Can you work these out from the model? Positions are in its coordinate system, mm. A direction names the side the tool comes from. Round coordinates to 2 decimals unless told otherwise and drop trailing zeros. Order: outer loops, then holes, each group sorted by start corner. A loop starts at its lowest first (then second) coordinate and runs counter-clockwise, first axis right, second up. Notation, with made-up numbers: M 89,-37 L 131,-37 A30 cw 131,-6 Z; hole C 55.5,5.25 d8. An arc over 180 degrees is marked long. Answer as a JSON object with one key per item and string values. Group by question number.
Autodesk Inventor part; units mm, degrees
ref_plane "Work Plane1" through (0, -29, 0) normal (0, 1, 0) x (-1, 0, 0)
ref_plane "Work Plane2" through (-18.485, -29, 0) normal (0, 0, 1) x (1, 0, 0)
ref_plane "YZ Plane" through (0, 0, 0) normal (1, 0, 0) x (0, 1, 0)
sketch "Sketch1" plane through (0, 0, 0) normal (0, 0, 1) x (1, 0, 0)
  circle A0 centre (0, 0) radius 28 construction
  circle A1 centre (0, 0) radius 29 construction
  circle A2 centre (0, 0) radius 28
  circle A3 centre (0, 0) radius 29
  line L0 (0, 0) -> (27.8935, 2.4404)
  line L1 (0, 0) -> (28, 0) construction
  line L2 (0, 0) -> (0, -29.5121)
  line L3 (0, -28) -> (0, -29)
  line L4 (27.8935, 2.4404) -> (28.8971, 2.4404)
  dimension "d0" = 56
  dimension "d1" = 58
  dimension "d2" = 5
revolve "Revolution1" add sketch "Sketch1" angle 360 about axis through (0, 0, 0) along (0, -1, 0) picked at (16.0405, -23.5642) contours A2 L4 A3 L2
sketch "Sketch2" plane through (0, 2.4404, 0) normal (0, 1, 0) x (1, 0, 0)
  line L0 (-0.5, -30) -> (0.5, -30)
  line L1 (0.5, -30) -> (0.5, 30)
  line L2 (0.5, 30) -> (-0.5, 30)
  line L3 (-0.5, 30) -> (-0.5, -30)
  line L4 (-0.5, -30) -> (0.5, 30) construction
  line L5 (0.5, -30) -> (-0.5, 30) construction
  line L6 (30, -0.5) -> (-30, -0.5)
  line L7 (-30, -0.5) -> (-30, 0.5)
  line L8 (-30, 0.5) -> (30, 0.5)
  line L9 (30, 0.5) -> (30, -0.5)
  circle A0 centre (0, 0) radius 28.8971
  line L10 (30, -0.5) -> (-30, 0.5) construction
  line L11 (-30, -0.5) -> (30, 0.5) construction
  point P0 (0.5, 0.5)
  point P1 (-0.5, 0.5)
  point P2 (-0.5, -0.5)
  point P3 (0.5, -0.5)
  dimension "d4" = 1
  dimension "d5" = 60
  dimension "d6" = 60
  dimension "d7" = 1
extrude "Extrusion1" cut sketch "Sketch2" against normal blind 15 contours L3 A0 L1 L0 | L3 L6 L1 A0 | L6 A0 L8 L3 | L3 L8 L1 L6 | L6 L7 L8 A0 | L1 L8 A0 L6 | A0 L8 L9 L6 | L3 A0 L1 L8 | L3 L2 L1 A0
ref_plane "Work Plane1" through (0, -29, 0) normal (0, 1, 0) x (-1, 0, 0)
sketch "Sketch3" plane through (0, -29, 0) normal (0, 1, 0) x (-1, 0, 0)
  arc A0 (-0.5, 28.8928) -> (-28.8928, 0.5) centre (0, 0) ccw
  arc A1 (-0.5, -26.1344) -> (0.5, -26.1344) centre (0, 0) ccw
  line L0 (0.5, -25.0201) -> (0.5, -26.1344)
  arc A2 (-0.5, -25.0201) -> (0.5, -25.0201) centre (0, 0) ccw
  line L1 (-0.5, -26.1344) -> (-0.5, -25.0201)
  circle A3 centre (0, 0) radius 26.1392
  line L2 (18.485, 18.4813) -> (-18.485, 18.4813)
  line L3 (-18.485, 18.4813) -> (-18.485, -18.4813)
  line L4 (-18.485, -18.4813) -> (18.485, -18.4813)
  line L5 (18.485, -18.4813) -> (18.485, 18.4813)
  line L6 (18.485, 18.4813) -> (-18.485, -18.4813) construction
  line L7 (-18.485, 18.4813) -> (18.485, -18.4813) construction
  dimension "d11" = 36.97
extrude "Extrusion2" add sketch "Sketch3" along normal up to surface contours L3 L2 L5 L4
sketch "Sketch4" plane through (0, -29, 0) normal (0, -1, 0) x (1, 0, 0)
  circle A0 centre (0, 0) radius 13.5
  dimension "d14" = 27
extrude "Extrusion3" cut sketch "Sketch4" against normal blind 10
fillet "Fillet1" radius 3 1 edges at (-13.5, -24.5306, 0)
fillet "Fillet2" radius 1 4 edges at (-19.7236, 2.4404, 19.7236) (-19.7236, 2.4404, -19.7236) (19.7236, 2.4404, -19.7236) (19.7236, 2.4404, 19.7236)
sketch "Sketch5" plane through (-18.485, -29, 18.4813) normal (0, 0, 1) x (1, 0, 0)
  line L0 (0, 0) -> (0, 16.4404) construction
  line L1 (0, 0) -> (1, 0) construction
  line L2 (1, 0) -> (1, 1) construction
  line L3 (1, 1) -> (0, 1) construction
  line L4 (0, 1) -> (0, 0) construction
  arc A0 (0, 16.4404) -> (36.97, 16.4404) centre (18.485, 29) ccw construction
  line L5 (0, 0) -> (0, 16.4404) construction
  line L6 (0, 0) -> (36.97, 0) construction
  line L7 (36.97, 0) -> (36.97, 16.4404) construction
  line L8 (1, 1) -> (35.97, 1) construction
  line L9 (35.97, 1) -> (35.97, 2.5) construction
  line L10 (35.97, 2.5) -> (1, 2.5) construction
  line L11 (1, 2.5) -> (1, 1) construction
  line L12 (1, 1) -> (35.97, 1)
  line L13 (35.97, 1) -> (35.97, 2.5)
  line L14 (35.97, 2.5) -> (1, 2.5)
  line L15 (1, 2.5) -> (1, 1)
  dimension "d19" = 1
  dimension "d20" = 1
  dimension "d21" = 34.97
  dimension "d22" = 1.5
extrude "Extrusion4" cut sketch "Sketch5" against normal blind 1
ref_plane "Work Plane2" through (-18.485, -29, 0) normal (0, 0, 1) x (1, 0, 0)
mirror "Mirror1" about plane through (-18.485, -29, 0) normal (0, 0, 1) of "Extrusion4"
properties part number "Socket"
Item 1: If we mould it in two halves opening along X, with no side actions, what happens to faces 1 (the face through (-18.485, -25, 0)), 2 (the face through (18.485, -25, 0)), 3 (the face through (-0.5, -5, 28))? For each: +X half, -X half, draft (parallel to the pull), parting line (faces both ways), or undercut.
Item 2: On a 3-axis mill with a long thin cutter (end or side, diameter ignored), from which of +Z, -Z, +X, -X, +Y, -Y can I reach the whole of each face in a straight line? I mean faces 4 (the face through (0, -25, 18.481)), 5 (the face through (0, -27, -17.481)), 6 (the face through (0, -27, 17.481)), 7 (the face through (0, -25, -18.481)). Say none if no direction works.
Item 3: Suppose I cut it at A-A, the plane y = -6. Write out the boundary of the cut face in (x, z), and give its area (3 significant figures).
Item 4: I'm going to push flat-ended pins straight in: pin 1 Ø1.1 at (y, z) = (-27, 18) entering from -X (3 decimals); pin 2 Ø0.8 at (x, z) = (0, 25.5) entering from +Y; pin 3 Ø5 at (x, y) = (-4.5, -17) entering from +Z. Where does each tip first touch, or does it pass through?
Item 5: Suppose I cut it at B-B, the plane y = -17. Write out the boundary of the cut face in (x, z) (3 decimals), and give its area (3 significant figures).
Item 6: I need wall thicknesses on line 1 (Z direction, x = 0, y = -28.25); line 2 (X direction, y = -27.8, z = 0) (3 decimals); line 3 (Z direction, x = 0, y = -27.25). Which ranges of each line are inside material? Lowest first, please.
Computed:
{
 "1": {"face 1": "-X half", "face 2": "+X half", "face 3": "undercut"},
 "2": {"face 4": "+Z, -Y", "face 5": "-Z", "face 6": "+Z", "face 7": "-Z, -Y"},
 "3": {"outline": "M -28.37,-0.5 A28.37 ccw -0.5,-28.37 L -0.5,-27.35 A27.35 cw -27.35,-0.5 Z; M -28.37,0.5 L -27.35,0.5 A27.35 cw -0.5,27.35 L -0.5,28.37 A28.37 ccw Z; M 0.5,-28.37 A28.37 ccw 28.37,-0.5 L 27.35,-0.5 A27.35 cw 0.5,-27.35 Z; M 0.5,27.35 A27.35 cw 27.35,0.5 L 28.37,0.5 A28.37 ccw 0.5,28.37 Z", "area": "175 mm^2"},
 "4": {"pin 1": "stops at x = -18.485", "pin 2": "stops at y = -12.56", "pin 3": "stops at z = 24.77"},
 "5": {"outline": "M -18.485,-18.481 L -14.507,-18.481 A23.495 ccw 14.507,-18.481 L 18.485,-18.481 L 18.485,-14.502 A23.495 ccw 18.485,14.502 L 18.485,18.481 L 14.507,18.481 A23.495 ccw -14.507,18.481 L -18.485,18.481 L -18.485,14.502 A23.495 ccw -18.485,-14.502 Z; hole C 0,0 d44.497", "area": "208 mm^2"},
 "6": {"line 1": "z = -18.48 to -13.5, 13.5 to 18.48", "line 2": "x = -18.485 to -13.5, 13.5 to 18.485", "line 3": "z = -17.48 to -13.5, 13.5 to 17.48"}
}
